Geometry: final body of the model. Coordinates: model frame, mm. A direction names the side the tool comes from. Give positions to 0.01 mm unless a question says otherwise; leave off trailing zeros. Order: outer loops, then holes, each group sorted by start corner. A loop starts at its lowest first (then second) coordinate and runs counter-clockwise, first axis right, second up. Notation, with made-up numbers: (-31.75, 69.5) -> (17.25, 69.5) arc R15 ccw to (17.25, 88.5) -> close; hole circle Ø9 at (-32.75, 32). An arc over 180 degrees is marked (long way). One line per question, with ' | ' between items. Start each with the question number.
(1) Set-up query: faces 5 (the face through (0, -2, -2)), 6 (the face through (2, 1.875, -2)). Return all of +Z, -Z, +X, -X, +Y, -Y with unobstructed straight access to the full face (end or side cutting, diameter ignored); none if empty.
(2) First-contact query: pin 1 Ø1 at (y, z) = (-1, -3) entering from +X. Flat tip, straight axial feed; report the tip coordinate or a pass-through.
(3) Section C-C (y = 0.9). Return loops of the section in (x, z).
(4) Mould query, pull axis X, two halves, no side actions, for faces 1 (the face through (0, 2, 2)), 2 (the face through (-0.45, -0.03, -1.43)), 3 (the face through (-3.04, 0.03, 3.32)), 4 (the face through (2, -1.875, 2)). Classes: +X half, -X half, draft (parallel to the pull), parting line (faces both ways), or undercut.
(5) Ray query, L1, parallel to X at y = 1.95, z = 0; L2, parallel to X at y = -0.45, z = 0; L3, parallel to Y at x = 0, z = 3 (3 decimals). Return the intervals inside material, ascending.
```python
from build123d import *

# Parameters (mm, degrees)
CHAMFER1_SIZE = 0.1


with BuildPart() as part:
    # Sketch2 → Revolve1 (revolve)
    with BuildSketch(Plane.XY, mode=Mode.PRIVATE) as revolve1_sk:
        Polygon((1.5, 2), (1.5, -2), (2.25, -2), (2.25, -1.875), (3.75, -1.875), (3.75, -2), (4.5, -2), (4.5, 2), (3.75, 2), (3.75, 1.875), (2.25, 1.875), (2.25, 2), align=None)
    revolve(revolve1_sk.sketch.rotate(Axis((0, -2, 0), (0, 1, 0)), 90), axis=Axis((0, -2, 0), (0, 1, 0)))

    # Chamfer1
    chamfer1_edges = [part.edges().sort_by_distance(p)[0] for p in [
        (0, 2, 4.5),
        (0, -2, 4.5),
        (0, -2, 1.5),
        (0, 2, 1.5),
    ]]
    chamfer(chamfer1_edges, length=CHAMFER1_SIZE)


solid = part.part
```
Response:
1) face 5: +Z, -Z, +X, -X, -Y | face 6: +Y
2) pin 1: stops at x = 3.74
3) outline: circle Ø9 at (0, 0); hole circle Ø3 at (0, 0)
4) face 1: draft | face 2: undercut | face 3: parting line | face 4: undercut
5) L1: x = -4.45 to -3.75, -2.25 to -1.55, 1.55 to 2.25, 3.75 to 4.45 | L2: x = -4.5 to -1.5, 1.5 to 4.5 | L3: y = -1.875 to 1.875
